from build123d import *

# Parameters (mm, degrees)
SKETCH_R        = 2.5
PAD_DEPTH       = 9
POCKET_DEPTH    = 53.001
POCKET001_DEPTH = 2


with BuildPart() as part:
    # Sketch → Pad (new body)
    with BuildSketch(Plane.XY):
        Polygon((-26.5, 28), (-18.5, 28), (-18.5, 23), (-13.5, 23), (-13.5, 28), (13.5, 28), (13.5, 23), (18.5, 23), (18.5, 28), (26.5, 28), (26.5, 20), (21.5, 20), (21.5, 15), (26.5, 15), (26.5, -15), (21.5, -15), (21.5, -20), (26.5, -20), (26.5, -28), (18.5, -28), (18.5, -23), (13.5, -23), (13.5, -28), (-13.5, -28), (-13.5, -23), (-18.5, -23), (-18.5, -28), (-26.5, -28), (-26.5, 15), (-21.5, 15), (-21.5, 20), (-26.5, 20), align=None)
        Circle(SKETCH_R, mode=Mode.SUBTRACT)
    extrude(amount=PAD_DEPTH)

    # Sketch001 (on Face15 of Pad) → Pocket (cut, through all)
    with BuildSketch(Plane.YZ.offset(26.5)):
        with BuildLine():
            ThreePointArc((-24, 9), (-23.12132, 6.87868), (-21, 6))
            Line((-21, 6), (-15, 6))
            Line((-15, 6), (-15, 9))
            Line((-15, 9), (-24, 9))
        make_face()
        with BuildLine():
            ThreePointArc((21, 6), (23.12132, 6.87868), (24, 9))
            Line((15, 9), (24, 9))
            Line((15, 6), (15, 9))
            Line((21, 6), (15, 6))
        make_face()
    extrude(amount=-POCKET_DEPTH, mode=Mode.SUBTRACT)

    # Sketch002 (on Face2 of Pocket) → Pocket001 (cut)
    with BuildSketch(Plane(origin=(0, 0, 0), x_dir=(1, 0, 0), z_dir=(0, 0, -1))):
        Polygon((2.75, -4.76314), (5.5, 0), (2.75, 4.76314), (-2.75, 4.76314), (-5.5, 0), (-2.75, -4.76314), align=None)
    extrude(amount=-POCKET001_DEPTH, mode=Mode.SUBTRACT)


solid = part.part
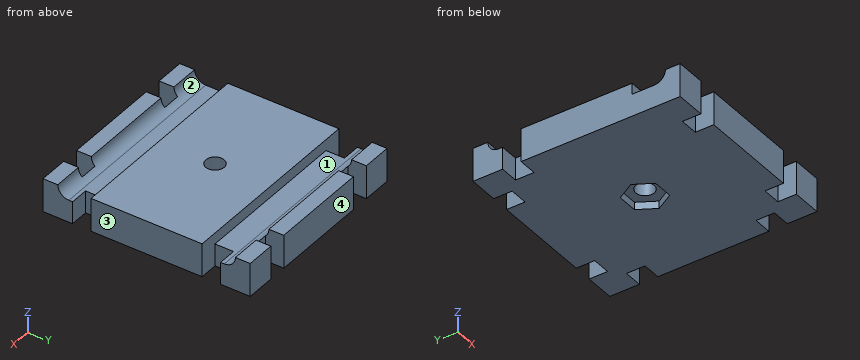
The listing builds one solid part. Answer for the finished solid, in the listing's coordinates (mm). Face numbers are marked on the shaded views. Give positions to 0.01 mm unless a question says otherwise; leave off trailing zeros. Loops run counter-clockwise (first coordinate to the right, second up) from the corner with the lowest first, then second, coordinate; pieces in that order, holes last. Notation, with made-up numbers: (3.5, 8) - (39.5, 8) arc R20 ccw to (39.5, 30) - close; hole circle Ø10 at (47.5, 70). An arc over 180 degrees is marked (long way). Answer as a JSON object with one key per item and string values.
1. A cutting plane is placed at A-A (z = 7.75). Give the number of separate pieces and of enclosed holes in the cut face, then the cut area to 3 significant figures.
Determined:
{"separate pieces": "7", "enclosed holes": "1", "area": "1,940 mm²"}
2. Flat-ended cylindrical pins translate along their axes: pin 1 Ø1.5 at (x, z) = (17, 4) entering from +Y; pin 2 Ø6.5 at (x, y) = (0, 0) entering from -Z; pin 3 Ø2.5 at (y, z) = (18.5, 3) entering from -X. Find the tip coordinate at first contact, or state that the pin passes through.
Determined:
{"pin 1": "y = 23", "pin 2": "z = 2", "pin 3": "x = -21.5"}
3. For a pull along Y with two mould halves and no side action, classify the marked faces 1, 2, 3 and 4 as pulls with the +Y half, pulls with the -Y half, needs draft (parallel to the pull), parting line crosses it, or undercut.
Determined:
{"face 1": "undercut", "face 2": "undercut", "face 3": "needs draft", "face 4": "pulls with the +Y half"}
4. A cutting plane is placed at D-D (x = 9). Write down the section's boundary in (y, z), then the cut area to 3 significant figures.
Determined:
{"outline": "(-28, 0) - (28, 0) - (28, 9) - (24, 9) arc R3 cw to (21, 6) - (15, 6) - (15, 9) - (-15, 9) - (-15, 6) - (-21, 6) arc R3 cw to (-24, 9) - (-28, 9) - close", "area": "454 mm²"}
5. Find the intervals of material crossed by L1, parallel to X at y = 26.5, z = 5.75; L2, parallel to Y at x = 13, z = 8.75; L3, parallel to Y at x = 0, z = 7.75, in increasing order. Write a range as [from, to].
Determined:
{"L1": "[-26.5, -18.5], [-13.5, 13.5], [18.5, 26.5]", "L2": "[-28, -23.99], [-15, 15], [23.99, 28]", "L3": "[-28, -23.73], [-15, -2.5], [2.5, 15], [23.73, 28]"}
6. A cutting plane is placed at B-B (x = 0). Write down the section's boundary in (y, z), then the cut area to 3 significant figures.
Determined:
{"outline": "(-28, 0) - (-4.76, 0) - (-4.76, 2) - (-2.5, 2) - (-2.5, 9) - (-15, 9) - (-15, 6) - (-21, 6) arc R3 cw to (-24, 9) - (-28, 9) - close; (2.5, 2) - (4.76, 2) - (4.76, 0) - (28, 0) - (28, 9) - (24, 9) arc R3 cw to (21, 6) - (15, 6) - (15, 9) - (2.5, 9) - close", "area": "400 mm²"}
